```python
from build123d import *

# Parameters (mm, degrees)
SKETCH1_W                   = 30
SKETCH1_H                   = 12
BOSS_EXTRUDE1_DEPTH         = 20
TAP_DRILL_FOR_M5X0_8_TAP1_D = 4.2
TAP_DRILL_FOR_M3X0_5_TAP1_D = 2.5
FILLET1_R                   = 0.5


with BuildPart() as part:
    # Sketch1 → Boss-Extrude1 (new body)
    with BuildSketch(Plane(origin=(0, 0, 0), x_dir=(1, 0, 0), z_dir=(0, 1, 0))):
        Rectangle(SKETCH1_W, SKETCH1_H)
    extrude(amount=BOSS_EXTRUDE1_DEPTH)

    # Tap Drill for M5x0.8 Tap1 (through all)
    with Locations(Plane(origin=(0, 0, 0), x_dir=(-1, 0, 0), z_dir=(0, -1, 0))):
        with Locations((0, 0)):
            Hole(TAP_DRILL_FOR_M5X0_8_TAP1_D / 2)

    # Tap Drill for M3x0.5 Tap1 (through all)
    with Locations(Plane.XY.offset(6)):
        with Locations((-10, 10), (10, 10)):
            Hole(TAP_DRILL_FOR_M3X0_5_TAP1_D / 2)

    # Fillet1
    fillet1_edges = [part.edges().sort_by_distance(p)[0] for p in [
        (-15, 10, -6),
        (15, 10, -6),
        (15, 10, 6),
        (-15, 10, 6),
    ]]
    fillet(fillet1_edges, radius=FILLET1_R)


solid = part.part
```
Input: part model. Units: mm. Frame: model coordinates. Coordinates: 2 decimals unless noted, no trailing zeros. Write each loop counter-clockwise with the first axis right and the second up, starting at its lowest first coordinate (ties: lowest second). Pieces come first, ordered by that corner, then holes.
1) Section C-C on x = 0. Output: boundary loops of the cut face in (y, z), and give its area (3 significant figures).
2) Section D-D on z = -3.5. Output: boundary loops of the cut face in (x, y), and give its area (3 significant figures).
3) Section A-A on y = 10. Output: boundary loops of the cut face in (x, z).
4) Material intervals for line 1 along Y through (x, z) = (10, -2.5); line 2 along Z through (x, y) = (0, 2); line 3 along Z through (x, y) = (1.75, 19.25), sorted ascending.
5) Section B-B on z = 0. Output: boundary loops of the cut face in (x, y).
6) Mould query, pull axis X, two halves, no side actions, for faces 1 (the cylindrical face through (10.921, 10.845, -0.084)), 2 (the cylindrical face through (2.003, 10.14, -0.631)), 3 (the flat face through (-15, 10, 0)), 4 (the flat face through (0, 20, -3)). Classes: pulls with the +X half, pulls with the -X half, needs draft (parallel to the pull), parting line crosses it, or undercut.
7) Pin query (flat end, axial travel): pin 1 Ø2.5 at (x, z) = (0, 0) entering from +Y. Return the tip coordinate at first contact, or that it passes through.
Check result:
1. outline: (0, -6) - (20, -6) - (20, -2.1) - (0, -2.1) - close; (0, 2.1) - (20, 2.1) - (20, 6) - (0, 6) - close
1. area: 156 mm2
2. outline: (-15, 0) - (15, 0) - (15, 20) - (-15, 20) - close; hole circle Ø2.5 at (-10, 10); hole circle Ø2.5 at (10, 10)
2. area: 590 mm2
3. outline: (-15, -5.5) arc R0.5 ccw to (-14.5, -6) - (-11.25, -6) - (-11.25, 6) - (-14.5, 6) arc R0.5 ccw to (-15, 5.5) - close; (-8.75, -6) - (8.75, -6) - (8.75, 6) - (-8.75, 6) - close; (11.25, -6) - (14.5, -6) arc R0.5 ccw to (15, -5.5) - (15, 5.5) arc R0.5 ccw to (14.5, 6) - (11.25, 6) - close; hole circle Ø4.2 at (0, 0)
4. line 1: y = 0 to 8.75, 11.25 to 20
4. line 2: z = -6 to -2.1, 2.1 to 6
4. line 3: z = -6 to -1.16, 1.16 to 6
5. outline: (-15, 0) - (-2.1, 0) - (-2.1, 20) - (-15, 20) - close; (2.1, 0) - (15, 0) - (15, 20) - (2.1, 20) - close; hole circle Ø2.5 at (-10, 10); hole circle Ø2.5 at (10, 10)
6. face 1: undercut
6. face 2: undercut
6. face 3: pulls with the -X half
6. face 4: needs draft
7. pin 1: passes through
